The model under review builds one solid part; all positions refer to its coordinate system, in mm. Face numbers are marked on the shaded views. A direction names the side the tool comes from. Round coordinates to 2 decimals unless told otherwise and drop trailing zeros. Write each loop counter-clockwise with the first axis right and the second up, starting at its lowest first coordinate (ties: lowest second). Pieces come first, ordered by that corner, then holes. Notation, with made-up numbers: (43.25, 82) - (91.25, 82) arc R25 ccw to (91.25, 113) - close; hole circle Ø8 at (2.5, 59). An arc over 180 degrees is marked (long way). Use one line per item in the form item = value.
from build123d import *

# Parameters (mm, degrees)
SKETCH1_R           = 1.190625
BOSS_EXTRUDE1_DEPTH = 12.7
SKETCH5_W           = 8.46735418
SKETCH5_H           = 3.96875
CUT_EXTRUDE2_DEPTH  = 48.176397098
FILLET1_R           = 2.54
FILLET2_START       = -2.835892255
FILLET2_DEPTH       = 12.592298151
FILLET2_2_DEPTH     = 13
CUT_EXTRUDE3_DEPTH  = 48.176397125
FILLET3_R           = 0.79375


with BuildPart() as part:
    # Sketch1 → Boss-Extrude1 (new body)
    with BuildSketch(Plane.XY):
        Polygon((2.943594104, -2.943594104), (2.943594104, 9.756405896), (-43.623760076, 9.756405896), (-43.623760076, -0.0889), (-5.523760076, -0.0889), (-2.669065971, -2.943594104), align=None)
        Circle(SKETCH1_R, mode=Mode.SUBTRACT)
    extrude(amount=BOSS_EXTRUDE1_DEPTH)

    # Sketch5 → Cut-Extrude2 (cut, through all)
    with BuildSketch(Plane.XZ.offset(2.943594104)):
        with Locations((-1.290082986, 10.715625)):
            Rectangle(SKETCH5_W, SKETCH5_H)
        with Locations((-1.290082986, 1.984375)):
            Rectangle(SKETCH5_W, SKETCH5_H)
    extrude(amount=-CUT_EXTRUDE2_DEPTH, mode=Mode.SUBTRACT)

    # Fillet1
    fillet1_edges = [part.edges().sort_by_distance(p)[0] for p in [
        (-2.669065971, -2.943594104, 6.35),
        (2.943594104, 9.756405896, 6.35),
        (2.943594104, -2.943594104, 6.35),
    ]]
    fillet(fillet1_edges, radius=FILLET1_R)

    # Fillet2: read off the stored shape, not the designer's step
    # Fillet2 outline → Fillet2 (add)
    with BuildSketch(Plane(origin=(0, 0, 0), x_dir=(1, 0, 0), z_dir=(0, 1, 0)).offset(FILLET2_START)):
        with BuildLine():
            ThreePointArc((-5.523760076, -11.90625), (-4.593824106, -9.66118597), (-2.348760076, -8.73125))
            Line((-2.348760076, -8.73125), (-5.523760076, -8.73125))
            Line((-5.523760076, -8.73125), (-5.523760076, -11.90625))
        make_face()
        with BuildLine():
            ThreePointArc((-2.348760076, -3.96875), (-4.593824106, -3.03881403), (-5.523760076, -0.79375))
            Line((-5.523760076, -0.79375), (-5.523760076, -3.96875))
            Line((-5.523760076, -3.96875), (-2.348760076, -3.96875))
        make_face()
    extrude(amount=FILLET2_DEPTH)

    # Fillet2 2 outline → Fillet2 2 (cut)
    with BuildSketch(Plane.XY):
        with BuildLine():
            ThreePointArc((-2.348760048, -2.835892163), (-2.92030771, -2.583707388), (-3.413014747, -2.199645328))
            Line((-3.413014747, -2.199645328), (-5.523760076, -0.0889))
            Line((-5.523760076, -0.0889), (-5.523760076, -2.835892255))
            Line((-5.523760076, -2.835892255), (-2.348760048, -2.835892163))
        make_face()
    extrude(amount=FILLET2_2_DEPTH, mode=Mode.SUBTRACT)

    # Sketch9 → Cut-Extrude3 (cut, through all)
    with BuildSketch(Plane(origin=(0, 9.756405896, 0), x_dir=(1, 0, 0), z_dir=(0, 1, 0))):
        with BuildLine():
            Line((-37.273760076, -3.7719), (-29.336260076, -3.7719))
            ThreePointArc((-29.336260076, -3.7719), (-26.758160076, -6.35), (-29.336260076, -8.9281))
            Line((-29.336260076, -8.9281), (-37.273760076, -8.9281))
            ThreePointArc((-37.273760076, -8.9281), (-39.851860076, -6.35), (-37.273760076, -3.7719))
        make_face()
        with BuildLine():
            Line((-21.398760076, -3.7719), (-13.461260076, -3.7719))
            ThreePointArc((-13.461260076, -3.7719), (-10.883160076, -6.35), (-13.461260076, -8.9281))
            Line((-13.461260076, -8.9281), (-21.398760076, -8.9281))
            ThreePointArc((-21.398760076, -8.9281), (-23.976860076, -6.35), (-21.398760076, -3.7719))
        make_face()
    extrude(amount=-CUT_EXTRUDE3_DEPTH, mode=Mode.SUBTRACT)

    # Fillet3
    fillet3_edges = [part.edges().sort_by_distance(p)[0] for p in [
        (-43.623760076, 4.833752948, 12.7),
        (-43.623760076, 4.833752948, 0),
        (-5.523760076, 4.833752948, 12.7),
        (-5.523760076, 4.833752948, 0),
    ]]
    fillet(fillet3_edges, radius=FILLET3_R - 0.0001)  # a hair under: the kernel refuses the full size


solid = part.part
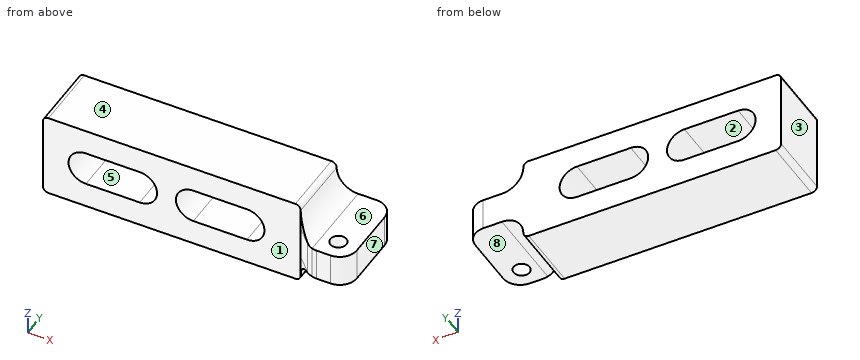
(1) Insertion check: P1, Ø5, axis at x = -38.5, z = 5, coming from the -Y side; P2, Ø1, axis at x = -12, y = -1, coming from the -Z side; P3, Ø2.5, axis at x = 1.5, y = 4.5, coming from the -Z side; P4, Ø1.6, axis at x = 0.5, y = 2, coming from the +Z side. Each pin has a flat end and moves straight along its axis. Give the tip position at first contact, or say it passes through.
Geometry results:
P1 = -0.09
P2 = through
P3 = 3.97
P4 = 8.73
(2) The part is to be moulded in two halves that separate along X. For the marked faces 1, 2 and 3, say which applies: +X half, -X half, draft (parallel to the pull), parting line (faces both ways), or undercut.
Geometry results:
face_1 = draft
face_2 = undercut
face_3 = -X half
(3) To check wall thickness, follow L1, parallel to X at y = 3.75, z = 6.5; L2, parallel to Z at x = -16.5, y = 7; L3, parallel to X at y = 3.5, z = 6.75. State the ranges of each line that lie inside material, in increasing order.
Geometry results:
L1 = -43.62 to -39.85, -26.76 to -23.97, -10.89 to 2.94
L2 = 0 to 3.77, 8.93 to 12.7
L3 = -43.62 to -39.82, -26.79 to -23.95, -10.91 to 2.94
(4) Add section D-D on z = 8.25. Write out the cut boundary in (x, y), then the cut area to 3 significant figures.
Geometry results:
outline = (-43.62, -0.09) - (-39.02, -0.09) - (-39.02, 9.76) - (-43.62, 9.76) - close; (-27.59, -0.09) - (-23.14, -0.09) - (-23.14, 9.76) - (-27.59, 9.76) - close; (-11.72, -0.09) - (-5.52, -0.09) - (-3.41, -2.2) arc R2.54 ccw to (-1.62, -2.94) - (0.4, -2.94) arc R2.54 ccw to (2.94, -0.4) - (2.94, 7.22) arc R2.54 ccw to (0.4, 9.76) - (-11.72, 9.76) - close; hole circle Ø2.38 at (0, 0)
area = 246 mm2
(5) Add section C-C on y = 5.25. Count the separate pieces of the cut face and the enclosed holes in it, then the cut area to 3 significant figures.
Geometry results:
separate_pieces = 1
enclosed_holes = 2
area = 404 mm2
(6) Add section B-B on x = -31. Write out the cut boundary in (y, z).
Geometry results:
outline = (-0.09, 0) - (9.76, 0) - (9.76, 3.77) - (-0.09, 3.77) - close; (-0.09, 8.93) - (9.76, 8.93) - (9.76, 12.7) - (-0.09, 12.7) - close
(7) Add section A-A on z = 6.35. Write out the cut boundary in (x, y), then the cut area to 3 significant figures.
Geometry results:
outline = (-43.62, -0.09) - (-39.85, -0.09) - (-39.85, 9.76) - (-43.62, 9.76) - close; (-26.76, -0.09) - (-23.98, -0.09) - (-23.98, 9.76) - (-26.76, 9.76) - close; (-10.88, -0.09) - (-5.52, -0.09) - (-3.41, -2.2) arc R2.54 ccw to (-1.62, -2.94) - (0.4, -2.94) arc R2.54 ccw to (2.94, -0.4) - (2.94, 7.22) arc R2.54 ccw to (0.4, 9.76) - (-10.88, 9.76) - close; hole circle Ø2.38 at (0, 0)
area = 213 mm2
(8) Machinability: for the marked faces 4, 5, 6, 7 and 8, which of the approach directions +Z, -Z, +X, -X, +Y, -Y give a long, thin tool a straight path to every point of the face, cutting with its end or side? Answer none if there is none.
Geometry results:
face_4 = +Z, +X, -X, +Y, -Y
face_5 = +Y, -Y
face_6 = +Z, +X, +Y, -Y
face_7 = +Z, -Z, +X, +Y, -Y
face_8 = -Z, +X, +Y, -Y
